from build123d import *

# Parameters (mm, degrees)
ESQUISSE1_R      = 3.4
EXTRUSION1_DEPTH = 224


with BuildPart() as part:
    # Esquisse1 → Extrusion1 (new body)
    with BuildSketch(Plane.XY.offset(20)):
        with BuildLine():
            Line((3.5, 16), (1.5, 16))
            ThreePointArc((1.5, 16), (0.439339828, 15.560660172), (0, 14.5))
            Line((0, 14.5), (0, 4))
            ThreePointArc((0, 4), (1.171572875, 1.171572875), (4, 0))
            Line((4, 0), (14.5, 0))
            ThreePointArc((14.5, 0), (15.560660172, 0.439339828), (16, 1.5))
            Line((16, 1.5), (16, 3.5))
            ThreePointArc((16, 3.5), (15.707106781, 4.207106781), (15, 4.5))
            Line((15, 4.5), (13.5, 4.5))
            ThreePointArc((13.5, 4.5), (13.146446609, 4.353553391), (13, 4))
            Line((13, 4), (13, 2.5))
            ThreePointArc((13, 2.5), (12.853553391, 2.146446609), (12.5, 2))
            ThreePointArc((12.5, 2), (10.732233047, 2.732233047), (10, 4.5))
            Line((10, 4.5), (10, 5.807611845))
            ThreePointArc((10, 5.807611845), (10.380602337, 7.721029006), (11.464466094, 9.343145751))
            Line((11.464466094, 9.343145751), (12.906854249, 10.785533906))
            ThreePointArc((12.906854249, 10.785533906), (14.528970994, 11.869397663), (16.442388155, 12.25))
            Line((16.442388155, 12.25), (23.557611845, 12.25))
            ThreePointArc((23.557611845, 12.25), (25.471029006, 11.869397663), (27.093145751, 10.785533906))
            Line((27.093145751, 10.785533906), (28.535533906, 9.343145751))
            ThreePointArc((28.535533906, 9.343145751), (29.619397663, 7.721029006), (30, 5.807611845))
            Line((30, 5.807611845), (30, 4.5))
            ThreePointArc((30, 4.5), (29.267766953, 2.732233047), (27.5, 2))
            ThreePointArc((27.5, 2), (27.146446609, 2.146446609), (27, 2.5))
            Line((27, 2.5), (27, 4))
            ThreePointArc((27, 4), (26.853553391, 4.353553391), (26.5, 4.5))
            Line((26.5, 4.5), (25, 4.5))
            ThreePointArc((25, 4.5), (24.292893219, 4.207106781), (24, 3.5))
            Line((24, 3.5), (24, 1.5))
            ThreePointArc((24, 1.5), (24.439339828, 0.439339828), (25.5, 0))
            Line((25.5, 0), (36, 0))
            ThreePointArc((36, 0), (38.828427125, 1.171572875), (40, 4))
            Line((40, 4), (40, 14.5))
            ThreePointArc((40, 14.5), (39.560660172, 15.560660172), (38.5, 16))
            Line((38.5, 16), (36.5, 16))
            ThreePointArc((36.5, 16), (35.792893219, 15.707106781), (35.5, 15))
            Line((35.5, 15), (35.5, 13.5))
            ThreePointArc((35.5, 13.5), (35.646446609, 13.146446609), (36, 13))
            Line((36, 13), (37.5, 13))
            ThreePointArc((37.5, 13), (37.853553391, 12.853553391), (38, 12.5))
            ThreePointArc((38, 12.5), (37.267766953, 10.732233047), (35.5, 10))
            Line((35.5, 10), (34.192388155, 10))
            ThreePointArc((34.192388155, 10), (32.278970994, 10.380602337), (30.656854249, 11.464466094))
            Line((30.656854249, 11.464466094), (29.214466094, 12.906854249))
            ThreePointArc((29.214466094, 12.906854249), (28.130602337, 14.528970994), (27.75, 16.442388155))
            Line((27.75, 16.442388155), (27.75, 23.557611845))
            ThreePointArc((27.75, 23.557611845), (28.130602337, 25.471029006), (29.214466094, 27.093145751))
            Line((29.214466094, 27.093145751), (30.656854249, 28.535533906))
            ThreePointArc((30.656854249, 28.535533906), (32.278970994, 29.619397663), (34.192388155, 30))
            Line((34.192388155, 30), (35.5, 30))
            ThreePointArc((35.5, 30), (37.267766953, 29.267766953), (38, 27.5))
            ThreePointArc((38, 27.5), (37.853553391, 27.146446609), (37.5, 27))
            Line((37.5, 27), (36, 27))
            ThreePointArc((36, 27), (35.646446609, 26.853553391), (35.5, 26.5))
            Line((35.5, 26.5), (35.5, 25))
            ThreePointArc((35.5, 25), (35.792893219, 24.292893219), (36.5, 24))
            Line((36.5, 24), (38.5, 24))
            ThreePointArc((38.5, 24), (39.560660172, 24.439339828), (40, 25.5))
            Line((40, 25.5), (40, 36))
            ThreePointArc((40, 36), (38.828427125, 38.828427125), (36, 40))
            Line((36, 40), (25.5, 40))
            ThreePointArc((25.5, 40), (24.439339828, 39.560660172), (24, 38.5))
            Line((24, 38.5), (24, 36.5))
            ThreePointArc((24, 36.5), (24.292893219, 35.792893219), (25, 35.5))
            Line((25, 35.5), (26.5, 35.5))
            ThreePointArc((26.5, 35.5), (26.853553391, 35.646446609), (27, 36))
            Line((27, 36), (27, 37.5))
            ThreePointArc((27, 37.5), (27.146446609, 37.853553391), (27.5, 38))
            ThreePointArc((27.5, 38), (29.267766953, 37.267766953), (30, 35.5))
            Line((30, 35.5), (30, 34.192388155))
            ThreePointArc((30, 34.192388155), (29.619397663, 32.278970994), (28.535533906, 30.656854249))
            Line((28.535533906, 30.656854249), (27.093145751, 29.214466094))
            ThreePointArc((27.093145751, 29.214466094), (25.471029006, 28.130602337), (23.557611845, 27.75))
            Line((23.557611845, 27.75), (16.442388155, 27.75))
            ThreePointArc((16.442388155, 27.75), (14.528970994, 28.130602337), (12.906854249, 29.214466094))
            Line((12.906854249, 29.214466094), (11.464466094, 30.656854249))
            ThreePointArc((11.464466094, 30.656854249), (10.380602337, 32.278970994), (10, 34.192388155))
            Line((10, 34.192388155), (10, 35.5))
            ThreePointArc((10, 35.5), (10.732233047, 37.267766953), (12.5, 38))
            ThreePointArc((12.5, 38), (12.853553391, 37.853553391), (13, 37.5))
            Line((13, 37.5), (13, 36))
            ThreePointArc((13, 36), (13.146446609, 35.646446609), (13.5, 35.5))
            Line((13.5, 35.5), (15, 35.5))
            ThreePointArc((15, 35.5), (15.707106781, 35.792893219), (16, 36.5))
            Line((16, 36.5), (16, 38.5))
            ThreePointArc((16, 38.5), (15.560660172, 39.560660172), (14.5, 40))
            Line((14.5, 40), (4, 40))
            ThreePointArc((4, 40), (1.171572875, 38.828427125), (0, 36))
            Line((0, 36), (0, 25.5))
            ThreePointArc((0, 25.5), (0.439339828, 24.439339828), (1.5, 24))
            Line((1.5, 24), (3.5, 24))
            ThreePointArc((3.5, 24), (4.207106781, 24.292893219), (4.5, 25))
            Line((4.5, 25), (4.5, 26.5))
            ThreePointArc((4.5, 26.5), (4.353553391, 26.853553391), (4, 27))
            Line((4, 27), (2.5, 27))
            ThreePointArc((2.5, 27), (2.146446609, 27.146446609), (2, 27.5))
            ThreePointArc((2, 27.5), (2.732233047, 29.267766953), (4.5, 30))
            Line((4.5, 30), (5.807611845, 30))
            ThreePointArc((5.807611845, 30), (7.721029006, 29.619397663), (9.343145751, 28.535533906))
            Line((9.343145751, 28.535533906), (10.785533906, 27.093145751))
            ThreePointArc((10.785533906, 27.093145751), (11.869397663, 25.471029006), (12.25, 23.557611845))
            Line((12.25, 23.557611845), (12.25, 16.442388155))
            ThreePointArc((12.25, 16.442388155), (11.869397663, 14.528970994), (10.785533906, 12.906854249))
            Line((10.785533906, 12.906854249), (9.343145751, 11.464466094))
            ThreePointArc((9.343145751, 11.464466094), (7.721029006, 10.380602337), (5.807611845, 10))
            Line((5.807611845, 10), (4.5, 10))
            ThreePointArc((4.5, 10), (2.732233047, 10.732233047), (2, 12.5))
            ThreePointArc((2, 12.5), (2.146446609, 12.853553391), (2.5, 13))
            Line((2.5, 13), (4, 13))
            ThreePointArc((4, 13), (4.353553391, 13.146446609), (4.5, 13.5))
            Line((4.5, 13.5), (4.5, 15))
            ThreePointArc((4.5, 15), (4.207106781, 15.707106781), (3.5, 16))
        make_face()
        with Locations(Location((20, 20, 0), (0, 0, 180))):
            Circle(ESQUISSE1_R, mode=Mode.SUBTRACT)
        with BuildLine():
            Line((1.8, 4), (1.8, 7.7))
            ThreePointArc((1.8, 7.7), (1.946446609, 8.053553391), (2.3, 8.2))
            Line((2.3, 8.2), (7.7, 8.2))
            ThreePointArc((7.7, 8.2), (8.053553391, 8.053553391), (8.2, 7.7))
            Line((8.2, 7.7), (8.2, 2.3))
            ThreePointArc((8.2, 2.3), (8.053553391, 1.946446609), (7.7, 1.8))
            Line((7.7, 1.8), (4, 1.8))
            ThreePointArc((4, 1.8), (2.444365081, 2.444365081), (1.8, 4))
        make_face(mode=Mode.SUBTRACT)
        with BuildLine():
            Line((36, 1.8), (32.3, 1.8))
            ThreePointArc((32.3, 1.8), (31.946446609, 1.946446609), (31.8, 2.3))
            Line((31.8, 2.3), (31.8, 7.7))
            ThreePointArc((31.8, 7.7), (31.946446609, 8.053553391), (32.3, 8.2))
            Line((32.3, 8.2), (37.7, 8.2))
            ThreePointArc((37.7, 8.2), (38.053553391, 8.053553391), (38.2, 7.7))
            Line((38.2, 7.7), (38.2, 4))
            ThreePointArc((38.2, 4), (37.555634919, 2.444365081), (36, 1.8))
        make_face(mode=Mode.SUBTRACT)
        with BuildLine():
            Line((38.2, 36), (38.2, 32.3))
            ThreePointArc((38.2, 32.3), (38.053553391, 31.946446609), (37.7, 31.8))
            Line((37.7, 31.8), (32.3, 31.8))
            ThreePointArc((32.3, 31.8), (31.946446609, 31.946446609), (31.8, 32.3))
            Line((31.8, 32.3), (31.8, 37.7))
            ThreePointArc((31.8, 37.7), (31.946446609, 38.053553391), (32.3, 38.2))
            Line((32.3, 38.2), (36, 38.2))
            ThreePointArc((36, 38.2), (37.555634919, 37.555634919), (38.2, 36))
        make_face(mode=Mode.SUBTRACT)
        with BuildLine():
            Line((4, 38.2), (7.7, 38.2))
            ThreePointArc((7.7, 38.2), (8.053553391, 38.053553391), (8.2, 37.7))
            Line((8.2, 37.7), (8.2, 32.3))
            ThreePointArc((8.2, 32.3), (8.053553391, 31.946446609), (7.7, 31.8))
            Line((7.7, 31.8), (2.3, 31.8))
            ThreePointArc((2.3, 31.8), (1.946446609, 31.946446609), (1.8, 32.3))
            Line((1.8, 32.3), (1.8, 36))
            ThreePointArc((1.8, 36), (2.444365081, 37.555634919), (4, 38.2))
        make_face(mode=Mode.SUBTRACT)
    extrude(amount=-EXTRUSION1_DEPTH)


solid = part.part
The listing builds one solid part. Answer for the finished solid, in the listing's coordinates (mm). A direction names the side the tool comes from. Round coordinates to 2 decimals unless told otherwise and drop trailing zeros. Write each loop counter-clockwise with the first axis right and the second up, starting at its lowest first coordinate (ties: lowest second). Pieces come first, ordered by that corner, then holes. Notation, with made-up numbers: M 57.5,75 L 104.5,75 A12 ccw 104.5,94 Z; hole C 71.25,65.25 d9. An arc over 180 degrees is marked long. Write each question's results on one line, items separated by ' | '. Start each with the question number.
(1) The part is cut by section C-C, the plane z = -37. Give the number of separate pieces and of enclosed holes in the cut face, and give its area (3 significant figures).
(2) Determine the mould class of faces 1 (the flat face through (9, 0, -90)), 2 (the flat face through (20, 27.75, -90)), 3 (the flat face through (12.25, 20, -90)), 4 (the flat face through (38.2, 6, -90)) for opening direction Y: +Y half, -Y half, draft (parallel to the pull), parting line (faces both ways), or undercut.
(3) Each of these flat-tipped pins is pushed along its axis until it touches: P1, Ø2, axis at y = 37.5, z = -70.5, coming from the -X side; P2, Ø1.6, axis at y = 37, z = -117, coming from the +X side (3 decimals); P3, Ø5, axis at x = 32.5, y = 16, coming from the -Z side; P4, Ø0.6, axis at x = 37.5, z = -98, coming from the +Y side. Where does it stop, or does it pass through?
(4) Find the intervals of material crossed by line 1 (Y direction, x = 20, z = -120.5); line 2 (Y direction, x = 15, z = -94.5); line 3 (X direction, y = 15.5, z = -147), in increasing order.
(5) For faces 5 (the cylindrical face through (1.141, 1.203, -90.432)), 6 (the cylindrical face through (7.746, 10.391, -90.432)), determine the directions among +Z, -Z, +X, -X, +Y, -Y from which every point of the face is accessible in a straight line to the end or side of a thin tool.
(6) The part is cut by section A-A, the plane y = 20. Write down the section's boundary in (x, z).
Worked answers:
1) separate pieces: 1 | enclosed holes: 5 | area: 657 mm²
2) face 1: -Y half | face 2: +Y half | face 3: undercut | face 4: undercut
3) P1: stops at x = 0.03 | P2: stops at x = 39.995 | P3: passes through | P4: stops at y = 39.82
4) line 1: y = 12.25 to 16.6, 23.4 to 27.75 | line 2: y = 0.09 to 4.5, 12.04 to 27.96, 35.5 to 39.91 | line 3: x = 0.38 to 4.37, 12.16 to 27.84, 35.63 to 39.62
5) face 5: +Z, -Z, -X, -Y | face 6: +Z, -Z
6) outline: M 12.25,-204 L 16.6,-204 L 16.6,20 L 12.25,20 Z; M 23.4,-204 L 27.75,-204 L 27.75,20 L 23.4,20 Z
